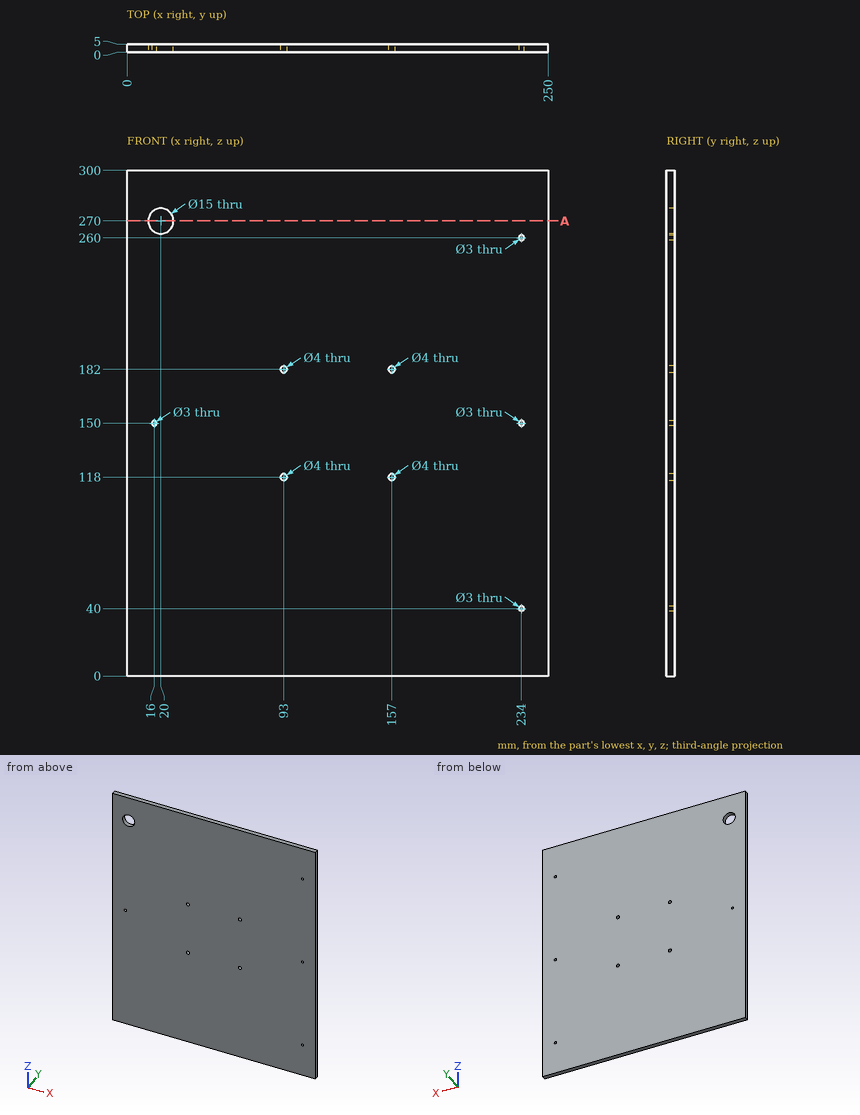
Study the drawing (mm; zero at the part's minimum x, y, z) and answer. Give positions to 0.01 mm unless a question says otherwise; leave off trailing zeros. Order: outer loops, then holes, each group sorted by start corner. A loop starts at its lowest first (then second) coordinate and runs counter-clockwise, first axis right, second up. Notation, with made-up numbers: (69, 18.5) -> (122, 18.5) arc R17 ccw to (122, 32.5) -> close; hole circle Ø8 at (78.5, -37.75). An arc over 180 degrees is marked (long way). Put each result on its own line as item: value.
Item 1: Given P1, Ø3.5, axis at x = 234, z = 40, coming from the +Y side, flat-ended and moving along its own axis, determine where the tip first touches the part or whether it passes through.
Established:
P1: stops at y = 5
Item 2: A cutting plane is placed at A-A on z = 270. Give the vertices of the cut face in (x, y).
Established:
outline: (0, 0) -> (12.5, 0) -> (12.5, 5) -> (0, 5) -> close; (27.5, 0) -> (250, 0) -> (250, 5) -> (27.5, 5) -> close
Item 3: Straight lines are drawn through the part: line 1 (X direction, y = 2.55, z = 182); line 2 (X direction, y = 1.45, z = 150); line 3 (Z direction, x = 93, y = 3.5). For each, find the intervals that lie inside material, in ascending order.
Established:
line 1: x = 0 to 91, 95 to 155, 159 to 250
line 2: x = 0 to 14.5, 17.5 to 232.5, 235.5 to 250
line 3: z = 0 to 116, 120 to 180, 184 to 300
